from build123d import *

# Parameters (mm, degrees)
BOSS_EXTRUDE1_DEPTH      = 13.5
BOSS_EXTRUDE2_DEPTH      = 18.5
BOSS_EXTRUDE3_DEPTH      = 5
SKETCH4_W                = 45.922011884
SKETCH4_H                = 20
BOSS_EXTRUDE4_DEPTH      = 13.5
SKETCH2_R                = 4
CUT_EXTRUDE1_DEPTH       = 282.548322307
SKETCH5_R                = 8
CUT_EXTRUDE2_DEPTH       = 4
SKETCH6_R                = 10
CUT_EXTRUDE3_DEPTH       = 8
BOSS_EXTRUDE5_DEPTH      = 13.5
CUT_EXTRUDE5_REACH       = 223.967
CUT_EXTRUDE5_END_RADIUS  = 45
SKETCH8_R                = 9
CUT_EXTRUDE6_REACH       = 223.967
SKETCH10_R               = 4
CUT_EXTRUDE7_START       = -4
SKETCH11_R               = 8
CUT_EXTRUDE7_DEPTH       = 4
SKETCH15_R               = 3
CUT_EXTRUDE8_DEPTH       = 224.567228
M6_CLEARANCE_HOLE1_D     = 6.4
CUT_EXTRUDE9_REACH       = 234.304
SKETCH20_R               = 4.5
CIRPATTERN1_COUNT        = 2
CUT_EXTRUDE10_REACH      = 284.756
CUT_EXTRUDE10_END_RADIUS = 10
SKETCH21_R               = 2.5
SKETCH22_R               = 11
CUT_EXTRUDE11_DEPTH      = 47


with BuildPart() as part:
    # Sketch1 → Boss-Extrude1 (new, symmetric)
    with BuildSketch(Plane(origin=(0, 0, 0), x_dir=(1, 0, 0), z_dir=(0, 1, 0))):
        with BuildLine():
            ThreePointArc((17.220754456, -41.574578963), (0, -45), (-17.220754456, -41.574578963))
            Line((-17.220754456, -41.574578963), (-22.961005942, -55.432771951))
            ThreePointArc((-22.961005942, -55.432771951), (0, -60), (22.961005942, -55.432771951))
            Line((22.961005942, -55.432771951), (17.220754456, -41.574578963))
        make_face()
    extrude(amount=BOSS_EXTRUDE1_DEPTH, both=True)

    # Sketch1<3> → Boss-Extrude2 (add, symmetric)
    with BuildSketch(Plane(origin=(0, 0, 0), x_dir=(1, 0, 0), z_dir=(0, 1, 0))):
        with BuildLine():
            ThreePointArc((19.134171618, -46.193976626), (0, -50), (-19.134171618, -46.193976626))
            Line((-19.134171618, -46.193976626), (-21.04758878, -50.813374288))
            ThreePointArc((-21.04758878, -50.813374288), (0, -55), (21.04758878, -50.813374288))
            Line((21.04758878, -50.813374288), (19.134171618, -46.193976626))
        make_face()
    extrude(amount=BOSS_EXTRUDE2_DEPTH, both=True)

    # Sketch3 → Boss-Extrude3 (add, symmetric)
    with BuildSketch(Plane.XZ):
        with BuildLine():
            Line((-22.961005942, 280), (-22.961005942, 55.432771951))
            ThreePointArc((-22.961005942, 55.432771951), (-20.481139434, 56.39612511), (-17.961005942, 57.248600555))
            Line((-17.961005942, 57.248600555), (-17.961005942, 260))
            Line((-17.961005942, 260), (17.961005942, 260))
            Line((17.961005942, 260), (17.961005942, 57.248600555))
            ThreePointArc((17.961005942, 57.248600555), (20.481139434, 56.39612511), (22.961005942, 55.432771951))
            Line((22.961005942, 55.432771951), (22.961005942, 280))
            Line((22.961005942, 280), (-22.961005942, 280))
        make_face()
    extrude(amount=BOSS_EXTRUDE3_DEPTH, both=True)

    # Sketch4 → Boss-Extrude4 (add, symmetric)
    with BuildSketch(Plane(origin=(0, 0, 0), x_dir=(1, 0, 0), z_dir=(0, 1, 0))):
        with Locations((0, -270)):
            Rectangle(SKETCH4_W, SKETCH4_H)
    extrude(amount=BOSS_EXTRUDE4_DEPTH, both=True)

    # Sketch2 → Cut-Extrude1 (cut, through all)
    with BuildSketch(Plane.XY):
        with Locations(Location((0, 0, 0), (0, 0, 180))):
            Circle(SKETCH2_R)
    extrude(amount=CUT_EXTRUDE1_DEPTH, mode=Mode.SUBTRACT)

    # Sketch5 → Cut-Extrude2 (cut)
    with BuildSketch(Plane(origin=(0, 0, 260), x_dir=(-1, 0, 0), z_dir=(0, 0, -1))):
        Circle(SKETCH5_R)
    extrude(amount=-CUT_EXTRUDE2_DEPTH, mode=Mode.SUBTRACT)

    # Sketch6 → Cut-Extrude3 (cut)
    with BuildSketch(Plane.XY.offset(280)):
        Circle(SKETCH6_R)
    extrude(amount=-CUT_EXTRUDE3_DEPTH, mode=Mode.SUBTRACT)

    # Sketch9 → Boss-Extrude5 (add, symmetric)
    with BuildSketch(Plane(origin=(0, 0, 0), x_dir=(1, 0, 0), z_dir=(0, 1, 0))):
        with BuildLine():
            Line((-22.961005942, -55.432771951), (-22.961005942, -68))
            Line((-22.961005942, -68), (22.961005942, -68))
            Line((22.961005942, -68), (22.961005942, -55.432771951))
            ThreePointArc((22.961005942, -55.432771951), (0, -60), (-22.961005942, -55.432771951))
        make_face()
    extrude(amount=BOSS_EXTRUDE5_DEPTH, both=True)

    # Cut-Extrude5: up to this cylinder (the profile starts outside it)
    cut_extrude5_end = Plane(origin=(0, 0, 0), z_dir=(0, -1, 0)) * Cylinder(CUT_EXTRUDE5_END_RADIUS, 538.934, mode=Mode.PRIVATE)
    # Sketch8 → Cut-Extrude5 (cut, up to the surface)
    with BuildSketch(Plane.XY.offset(60), mode=Mode.PRIVATE) as cut_extrude5_sk1:
        Circle(SKETCH8_R)
    cut_extrude5_tool1 = extrude(cut_extrude5_sk1.sketch, amount=-CUT_EXTRUDE5_REACH, mode=Mode.PRIVATE) - cut_extrude5_end
    add(cut_extrude5_tool1.solids().sort_by_distance((0, 0, 60))[0], mode=Mode.SUBTRACT)

    # Sketch10 → Cut-Extrude6 (cut, up to next)
    with BuildSketch(Plane.XY.offset(60), mode=Mode.PRIVATE) as cut_extrude6_sk1:
        with Locations(Location((0, 0, 0), (0, 0, 180))):
            Circle(SKETCH10_R)
    cut_extrude6_tool1 = extrude(cut_extrude6_sk1.sketch, amount=CUT_EXTRUDE6_REACH, mode=Mode.PRIVATE) & part.part
    add(cut_extrude6_tool1.solids().sort_by_distance((0, 0, 60))[0], mode=Mode.SUBTRACT)

    # Sketch11 → Cut-Extrude7 (cut)
    with BuildSketch(Plane.XY.offset(68).offset(CUT_EXTRUDE7_START)):
        with Locations(Location((0, 0, 0), (0, 0, 180))):
            Circle(SKETCH11_R)
    extrude(amount=CUT_EXTRUDE7_DEPTH, mode=Mode.SUBTRACT)

    # Sketch15 → Cut-Extrude8 (cut)
    with BuildSketch(Plane.XY.offset(280)):
        with Locations((-12.167449647, -9.762846361)):
            Circle(SKETCH15_R)
        with Locations((12.167449647, 9.762846361)):
            Circle(SKETCH15_R)
    extrude(amount=-CUT_EXTRUDE8_DEPTH, mode=Mode.SUBTRACT)

    # Sketch17 → M2 Tapped Hole1 (revolve, cut)
    with BuildSketch(Plane(origin=(22.961005942, 9.762846361, 272), x_dir=(0, 0, -1), z_dir=(0, 1, 0))):
        Polygon((0, 0), (0, 10.480688495), (0.8, 10), (0.8, 0), align=None)
    m2_tapped_hole1 = revolve(axis=Axis((29.311005942, 9.762846361, 272), (-1, 0, 0)), mode=Mode.SUBTRACT)

    # M6 Clearance Hole1 (through all)
    with Locations(Plane(origin=(0, 18.5, 0), x_dir=(1, 0, 0), z_dir=(0, 1, 0))):
        with Locations((13.587999868, -50.71110588), (-13.587999868, -50.71110588)):
            Hole(M6_CLEARANCE_HOLE1_D / 2)

    # Sketch20 → Cut-Extrude9 (cut, up to next)
    with BuildSketch(Plane.XY.offset(272), mode=Mode.PRIVATE) as cut_extrude9_sk1:
        Circle(SKETCH20_R)
    cut_extrude9_tool1 = extrude(cut_extrude9_sk1.sketch, amount=-CUT_EXTRUDE9_REACH, mode=Mode.PRIVATE) & part.part
    add(cut_extrude9_tool1.solids().sort_by_distance((0, 0, 272))[0], mode=Mode.SUBTRACT)

    # CirPattern1: M2 Tapped Hole1 ×2 about axis
    cirpattern1_axis = Axis((0, 0, 68), (0, 0, 1))
    for i in range(1, CIRPATTERN1_COUNT):
        add(m2_tapped_hole1.rotate(cirpattern1_axis, i * 360 / CIRPATTERN1_COUNT), mode=Mode.SUBTRACT)

    # Cut-Extrude10: up to this cylinder (the profile starts outside it)
    cut_extrude10_end = Plane(origin=(0, 0, 275), z_dir=(0, 0, 1)) * Cylinder(CUT_EXTRUDE10_END_RADIUS, 590.512, mode=Mode.PRIVATE)
    # Sketch21 → Cut-Extrude10 (cut, up to the surface)
    with BuildSketch(Plane(origin=(0, 13.5, 0), x_dir=(1, 0, 0), z_dir=(0, 1, 0)), mode=Mode.PRIVATE) as cut_extrude10_sk1:
        with Locations(Location((0, -275, 0), (0, 0, 270))):
            Circle(SKETCH21_R)
    cut_extrude10_tool1 = extrude(cut_extrude10_sk1.sketch, amount=-CUT_EXTRUDE10_REACH, mode=Mode.PRIVATE) - cut_extrude10_end
    add(cut_extrude10_tool1.solids().sort_by_distance((0, 13.5, 275))[0], mode=Mode.SUBTRACT)

    # Sketch22 → Cut-Extrude11 (cut)
    with BuildSketch(Plane.XY):
        with Locations(Location((0, 0, 0), (0, 0, 180))):
            Circle(SKETCH22_R)
    extrude(amount=CUT_EXTRUDE11_DEPTH, mode=Mode.SUBTRACT)


solid = part.part
Build history of the part. All positions in model axes, mm. A direction names the side the tool comes from. Coordinates: 2 decimals unless noted, no trailing zeros. Write each loop counter-clockwise with the first axis right and the second up, starting at its lowest first coordinate (ties: lowest second). Pieces come first, ordered by that corner, then holes.
(1) Cut at A-A on y = -15.5. List the corners of the cut face in (x, z).
(2) Drill centre lines: line 1 (Z direction, x = 15, y = 0.5); line 2 (Z direction, x = 13, y = 0); line 3 (Y direction, x = 0, z = 54). Where is each one in solid material? Low to high.
(3) Cut at B-B on z = 111.5. List the corners of the cut face in (x, y).
(4) Cut at C-C on x = 0. State how many separate pieces and enclosed holes the cut face has, and give its area (4 significant figures).
(5) 3-axis set-ups, long thin cutter, end or side, ignore diameter. For faces 5 (the cylindrical face through (-18.68, -15.96, 51.73)), 6 (the cylindrical face through (1.73, 7.81, 65.97)), 7 (the cylindrical face through (-0.59, 4.46, 268.06)): which of +Z, -Z, +X, -X, +Y, -Y reach the whole face in a straight line?
(6) Pin check, flat tips, straight feed: pin 1 Ø22 at (x, z) = (-11.5, 269.5) entering from +Y; pin 2 Ø5.5 at (x, y) = (12.17, 9.76) entering from -Z; pin 3 Ø5 at (x, y) = (12.17, 9.76) entering from +Z; pin 4 Ø1.5 at (x, z) = (16.5, 166) entering from +Y. Stop position of each tip, or through.
(7) Cut at D-D on z = 275. List the corners of the cut face in (x, y), and give its area (3 significant figures).
(8) Mould opens along X. For faces 1 (the flat face through (12, 10, 55.433)), 2 (the flat face through (4.3, -2.1, 272)), 3 (the flat face through (-22.961, 0, 166)), 4 (the flat face through (0, 13.5, 270)) say: pulls with the +X half, pulls with the -X half, needs draft (parallel to the pull), parting line crosses it, or undercut.
Working result:
1. outline: (-21.05, 50.81) - (-19.13, 46.19) arc R50 cw to (-14.81, 47.76) arc R3.2 cw to (-16.2, 52.56) arc R55 ccw to start; (-12.25, 53.62) arc R3.2 cw to (-11.05, 48.76) arc R50 cw to (11.05, 48.76) arc R3.2 cw to (12.25, 53.62) arc R55 ccw to start; (14.81, 47.76) arc R50 cw to (19.13, 46.19) - (21.05, 50.81) arc R55 ccw to (16.2, 52.56) arc R3.2 cw to start
2. line 1: z = 42.43 to 47.84, 53.58 to 68, 260 to 280
2. line 2: z = 43.08 to 47.57, 53.86 to 68, 260 to 280
2. line 3: y = -18.5 to -9, 9 to 18.5
3. outline: (-22.96, -5) - (-17.96, -5) - (-17.96, 5) - (-22.96, 5) - close; (17.96, -5) - (22.96, -5) - (22.96, 5) - (17.96, 5) - close
4. separate pieces: 5
4. enclosed holes: 0
4. area: 523.5 mm2
5. face 5: +Z, -X, -Y
5. face 6: none
5. face 7: +Z
6. pin 1: stops at y = 13.5
6. pin 2: stops at z = 42.45
6. pin 3: stops at z = 55.43
6. pin 4: passes through
7. outline: (-22.96, -13.5) - (22.96, -13.5) - (22.96, 13.5) - (2.5, 13.5) - (2.5, 9.68) arc R10 cw (long way) to (-2.5, 9.68) - (-2.5, 13.5) - (-22.96, 13.5) - close; hole circle Ø6 at (-12.17, -9.76); hole circle Ø6 at (12.17, 9.76)
7. area: 851 mm2
8. face 1: undercut
8. face 2: undercut
8. face 3: pulls with the -X half
8. face 4: needs draft
